Here's the drawing with two shaded views (mm, measured from the low corner). I have some questions. A direction names the side the tool comes from. Round coordinates to 2 decimals unless told otherwise and drop trailing zeros. Order: outer loops, then holes, each group sorted by start corner. A loop starts at its lowest first (then second) coordinate and runs counter-clockwise, first axis right, second up. Notation, with made-up numbers: (-24.75, 55) -> (20.25, 55) arc R9 ccw to (20.25, 71) -> close; hole circle Ø11 at (69.25, 51). An arc over 180 degrees is marked (long way). Use a Markdown table: item, result. Add a question column.
Q1. I'm going to push flat-ended pins straight in: pin 1 Ø3 at (x, z) = (36.455, 5.715) entering from -Y; pin 2 Ø8 at (y, z) = (13.5, 15.5) entering from -X; pin 3 Ø1.3 at (y, z) = (6.5, 43) entering from +X (3 decimals); pin 4 Ø1.5 at (x, z) = (31.5, 7.5) entering from +Y. Where does each tip first touch, or does it pass through?
Q2. For the marked faces 1 and 2, which set-ups out of +Z, -Z, +X, -X, +Y, -Y let a thin tool reach every point of the face, with its end or its side?
Q3. I need wall thicknesses on line 1 along Y through (x, z) = (15, 10); line 2 along Z through (x, y) = (17.5, 15); line 3 along Y through (x, z) = (24, 15). Which ranges of each line are inside material? Lowest first, please. Write a range as [from, to].
Q4. If we section it at A-A on y = 19: List the corners of the cut face in (x, z) for me (3 decimals), plus the area to 3 significant figures.
Q5. If we section it at C-C on z = 11.5: List the corners of the cut face in (x, y) for me.
Q6. If we section it at B-B on x = 13: List the corners of the cut face in (y, z) for me, plus the area to 3 significant figures.
Q7. If we section it at D-D on y = 4: List the corners of the cut face in (x, z) for me (3 decimals), plus the area to 3 significant figures.
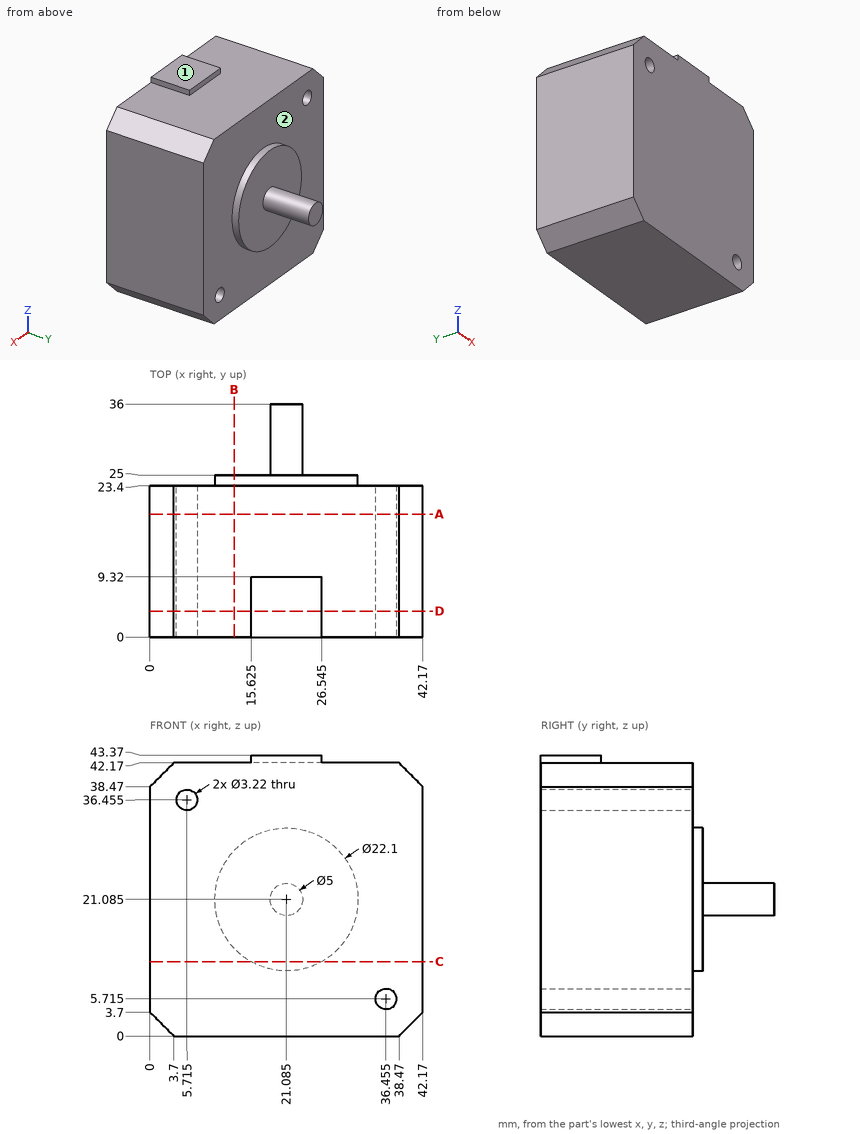
Answer below:
| question | item | result |
|---|---|---|
| 1 | pin 1 | through |
| 1 | pin 2 | x = 0 |
| 1 | pin 3 | x = 26.545 |
| 1 | pin 4 | y = 23.4 |
| 2 | face 1 | +Z, +X, -X, +Y, -Y |
| 2 | face 2 | +Y |
| 3 | line 1 | [0, 23.4] |
| 3 | line 2 | [0, 42.17] |
| 3 | line 3 | [0, 25] |
| 4 | outline | (0, 3.7) -> (3.7, 0) -> (38.47, 0) -> (42.17, 3.7) -> (42.17, 38.47) -> (38.47, 42.17) -> (3.7, 42.17) -> (0, 38.47) -> close; hole circle Ø3.22 at (5.715, 36.455); hole circle Ø3.22 at (36.455, 5.715) |
| 4 | area | 1,730 mm² |
| 5 | outline | (0, 0) -> (42.17, 0) -> (42.17, 23.4) -> (26.58, 23.4) -> (26.58, 25) -> (15.59, 25) -> (15.59, 23.4) -> (0, 23.4) -> close |
| 6 | outline | (0, 0) -> (23.4, 0) -> (23.4, 13.55) -> (25, 13.55) -> (25, 28.62) -> (23.4, 28.62) -> (23.4, 42.17) -> (0, 42.17) -> close |
| 6 | area | 1,010 mm² |
| 7 | outline | (0, 3.7) -> (3.7, 0) -> (38.47, 0) -> (42.17, 3.7) -> (42.17, 38.47) -> (38.47, 42.17) -> (26.545, 42.17) -> (26.545, 43.37) -> (15.625, 43.37) -> (15.625, 42.17) -> (3.7, 42.17) -> (0, 38.47) -> close; hole circle Ø3.22 at (5.715, 36.455); hole circle Ø3.22 at (36.455, 5.715) |
| 7 | area | 1,750 mm² |
